```python
from build123d import *

# Parameters (mm, degrees)
F1_DEPTH      = 30
F1_DEPTH_BACK = 30
F3_W          = 20
F3_H          = 96
F4_DEPTH      = 30
F6_DEPTH      = 40
F8_DEPTH      = 90
F9_DEPTH      = 60.001
F11_DEPTH     = 25
F12_R         = 9.99999
F13_R         = 5
F14_DEPTH     = 120.001
F15_R         = 5
F16_DEPTH     = 40.001
F17_SIZE2     = 2.5
F17_SIZE      = 3.5
F18_R         = 7
F19_DEPTH     = 60.001


# Not quite as in the source:
# - a fillet or chamfer is up to 0.001 mm smaller than in the source, because OpenCascade refuses the exact size


with BuildPart() as f1:
    # F0 (on Front) → F1 (new body, two sides)
    with BuildSketch(Plane.XZ) as f1_sk:
        Polygon((-80, 40), (-120, 40), (-120, -20), (-50, -20), (-50, 20), align=None)
    extrude(amount=F1_DEPTH)
    extrude(f1_sk.sketch, amount=-F1_DEPTH_BACK)

    # F3 (on face) → F4 (cut)
    with BuildSketch(Plane.YZ.offset(-50)):
        Rectangle(F3_W, F3_H)
    extrude(amount=-F4_DEPTH, mode=Mode.SUBTRACT)

    # F5 (on face) → F6 (join)
    with BuildSketch(Plane.YZ.offset(-80)):
        with BuildLine():
            Line((-30, 20), (-10, 20))
            Line((-10, 20), (-10, 70))
            ThreePointArc((-10, 70), (-20, 80), (-30, 70))
            Line((-30, 70), (-30, 20))
        make_face()
        with BuildLine():
            Line((10, 50), (10, 20))
            Line((10, 20), (30, 20))
            Line((30, 20), (30, 50))
            ThreePointArc((30, 50), (20, 60), (10, 50))
        make_face()
    extrude(amount=-F6_DEPTH)

    # F7 (on Right) → F8 (join)
    with BuildSketch(Plane.YZ):
        Polygon((-20, 5), (-30, 5), (-30, -5), (-20, -5), (-20, -20), (20, -20), (20, -5), (30, -5), (30, 5), (20, 5), (20, 20), (-20, 20), align=None)
    extrude(amount=-F8_DEPTH)

    # F2 (on face) → F9 (cut, through all)
    with BuildSketch(Plane.XZ.offset(30)):
        Polygon((-90, 10), (-128, 10), (-128, -28), (-60, -28), (-60, -10), align=None)
    extrude(amount=-F9_DEPTH, mode=Mode.SUBTRACT)

    # F10 (on face) → F11 (cut)
    with BuildSketch(Plane.YZ):
        Polygon((0, 14.1421356237), (-14.1421356237, 0), (0, -14.1421356237), (14.1421356237, 0), align=None)
    extrude(amount=-F11_DEPTH, mode=Mode.SUBTRACT)

    # F12 (radius 10 in the source; OpenCascade refuses exactly that, so slightly less here)
    f12_edges = [f1.edges().sort_by_distance(p)[0] for p in [
        (-25, 20, 20),
        (-25, -20, 20),
    ]]
    fillet(f12_edges, radius=F12_R)

    # F13 (on face) → F14 (cut, through all)
    with BuildSketch(Plane.YZ):
        with Locations((-7, -20)):
            Circle(F13_R)
        with Locations((7, -20)):
            Circle(F13_R)
    extrude(amount=-F14_DEPTH, mode=Mode.SUBTRACT)

    # F15 (on face) → F16 (cut, through all)
    with BuildSketch(Plane.YZ.offset(-80)):
        with Locations((-20, 70)):
            Circle(F15_R)
        with Locations((20, 50)):
            Circle(F15_R)
    extrude(amount=-F16_DEPTH, mode=Mode.SUBTRACT)

    # F17
    f17_edges = [f1.edges().sort_by_distance(p)[0] for p in [
        (-120, 0, 10),
    ]]
    chamfer(f17_edges, length=F17_SIZE, length2=F17_SIZE2)

    # F18 (on face) → F19 (cut, through all)
    with BuildSketch(Plane.XZ.offset(30)):
        with Locations((-105, 10)):
            Circle(F18_R)
    extrude(amount=-F19_DEPTH, mode=Mode.SUBTRACT)


solid = f1.part
```
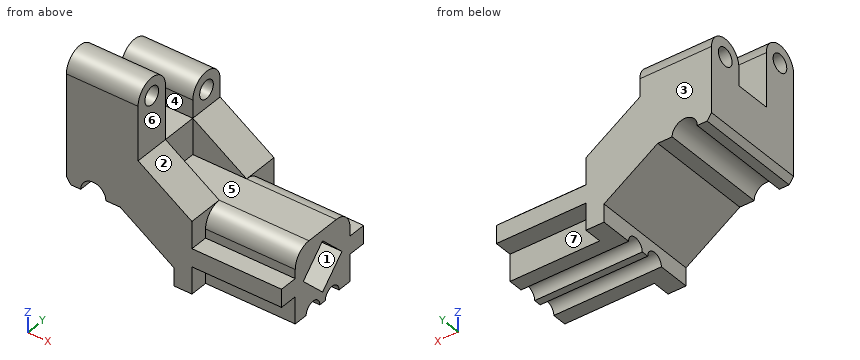
The model under review builds one solid part; all positions refer to its coordinate system, in mm. Face numbers are marked on the shaded views. A direction names the side the tool comes from. Coordinates: 2 decimals unless noted, no trailing zeros. Order: outer loops, then holes, each group sorted by start corner. A loop starts at its lowest first (then second) coordinate and runs counter-clockwise, first axis right, second up. Notation, with made-up numbers: (-16.75, -40) -> (2.25, -40) arc R31 cw to (2.25, -12) -> close; hole circle Ø10 at (46, -2.5). An arc over 180 degrees is marked (long way). Answer in a Markdown table with one row per item. Add a question column.
Item 1: Mouldability with a two-part tool opening along Y and no side actions: class the marked faces 1, 2 and 3 as +Y half, -Y half, draft (parallel to the pull), parting line (faces both ways), or undercut.
Item 2: Machinability: for the marked faces 4, 5, 6 and 7, which of the approach directions +Z, -Z, +X, -X, +Y, -Y give a long, thin tool a straight path to every point of the face, cutting with its end or side? Answer none if there is none.
Item 3: Clearance check with flat-ended pins moving along their axes: pin 1 (10 mm diameter, centred on x = -33.5, y = 17, fed in from +Z); pin 2 (2 mm diameter, centred on x = -43.5, y = 7.5, fed in from -Z); pin 3 (22 mm diameter, centred on y = 20.5, z = 53, fed in from +X). State where each tip first meets the part, or that it passes through.
Item 4: We need section B-B on z = 42. Write out the cut boundary in (x, y).
Item 5: We need section A-A on x = -105. Write out the cut boundary in (y, z).
Item 6: We need section C-C on x = -41.5. Write out the cut boundary in (y, z), plus the area to 3 significant figures.
Item 7: To check wall thickness, follow probe 1 along Y at (x, z) = (-77, 24.5); probe 2 along Z at (x, y) = (-106, -20); probe 3 along Z at (x, y) = (-96, 20). State the ranges of each line that lie inside material, in increasing order.
Item 8: We need section D-D on x = -9.5. Write out the cut boundary in (y, z), plus the area to 3 significant figures.
Final values:
| question | item | result |
|---|---|---|
| 1 | face 1 | undercut |
| 1 | face 2 | draft |
| 1 | face 3 | +Y half |
| 2 | face 4 | +Z, +X, -X |
| 2 | face 5 | +Z, +X |
| 2 | face 6 | +Z, +X, +Y, -Y |
| 2 | face 7 | -Z, +X, +Y |
| 3 | pin 1 | stops at z = 19.8 |
| 3 | pin 2 | stops at z = -15.23 |
| 3 | pin 3 | stops at x = -80 |
| 4 | outline | (-120, -30) -> (-80, -30) -> (-80, -10) -> (-120, -10) -> close; (-120, 10) -> (-80, 10) -> (-80, 30) -> (-120, 30) -> close |
| 5 | outline | (-30, 17) -> (30, 17) -> (30, 50) arc R10 ccw to (10, 50) -> (10, 40) -> (-10, 40) -> (-10, 70) arc R10 ccw to (-30, 70) -> close; hole circle Ø10 at (-20, 70); hole circle Ø10 at (20, 50) |
| 6 | outline | (-30, -5) -> (-20, -5) -> (-20, -20) -> (-12, -20) arc R5 cw to (-2, -20) -> (2, -20) arc R5 cw to (12, -20) -> (20, -20) -> (20, -5) -> (30, -5) -> (30, 5) -> (20, 5) -> (20, 10) arc R10 ccw to (10, 20) -> (-10, 20) arc R10 ccw to (-20, 10) -> (-20, 5) -> (-30, 5) -> close |
| 6 | area | 1,680 mm2 |
| 7 | probe 1 | y = -30 to -10, 10 to 30 |
| 7 | probe 2 | z = 16.93 to 65, 75 to 80 |
| 7 | probe 3 | z = 10 to 45, 55 to 60 |
| 8 | outline | (-30, -5) -> (-20, -5) -> (-20, -20) -> (-12, -20) arc R5 cw to (-2, -20) -> (2, -20) arc R5 cw to (12, -20) -> (20, -20) -> (20, -5) -> (30, -5) -> (30, 5) -> (20, 5) -> (20, 10) arc R10 ccw to (10, 20) -> (-10, 20) arc R10 ccw to (-20, 10) -> (-20, 5) -> (-30, 5) -> close; hole (-14.14, 0) -> (0, -14.14) -> (14.14, 0) -> (0, 14.14) -> close |
| 8 | area | 1,280 mm2 |
